For this review, take the finished solid that the model builds, in its own axes (mm). Give positions to 0.01 mm unless a question says otherwise; leave off trailing zeros. Loops run counter-clockwise (first coordinate to the right, second up) from the corner with the lowest first, then second, coordinate; pieces in that order, holes last.
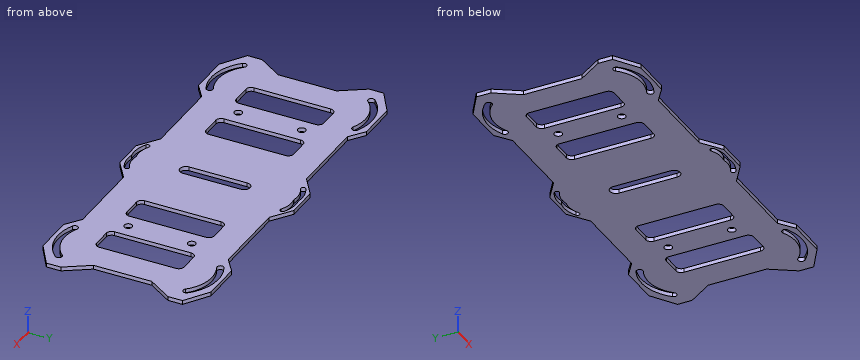
```python
from build123d import *

# Parameters (mm, degrees)
SCHIZZO1_R                   = 1.5
ESTRUSIONE_ESTRUSIONE1_DEPTH = 0.75


with BuildPart() as part:
    # Schizzo1 → Estrusione-Estrusione1 (new body, symmetric)
    with BuildSketch(Plane.XY):
        Polygon((-43.5, -27.5), (-13.615232638, -27.5), (-5.964504028, -32.859521299), (5.964504028, -32.859521299), (13.615232638, -27.5), (43.5, -27.5), (49.293787181, -31.722358535), (64.293787181, -31.722358535), (73.508072858, -25.714285677), (73.508072858, -20.214285677), (67.5, -11), (67.5, 11), (73.508072858, 20.214285677), (73.508072858, 25.714285677), (64.293787181, 31.722358535), (49.293787181, 31.722358535), (43.5, 27.5), (13.615232638, 27.5), (5.964504028, 32.859521299), (-5.964504028, 32.859521299), (-13.615232638, 27.5), (-43.5, 27.5), (-49.293787181, 31.722358535), (-64.293787181, 31.722358535), (-73.508072858, 25.714285677), (-73.508072858, 20.214285677), (-67.5, 11), (-67.5, -11), (-73.508072858, -20.214285677), (-73.508072858, -25.714285677), (-64.293787181, -31.722358535), (-49.293787181, -31.722358535), align=None)
        with BuildLine():
            ThreePointArc((-48.754479002, -28.623738791), (-59.172775767, -30.009764998), (-68.405644393, -24.988200197))
            ThreePointArc((-68.405644393, -24.988200197), (-68.356417198, -23.226138607), (-66.594355607, -23.275365801))
            ThreePointArc((-66.594355607, -23.275365801), (-58.719274878, -27.558458065), (-49.83309536, -26.376261209))
            ThreePointArc((-49.83309536, -26.376261209), (-48.17004839, -26.960691821), (-48.754479002, -28.623738791))
        make_face(mode=Mode.SUBTRACT)
        with Locations((-40.191447808, -12)):
            Circle(SCHIZZO1_R, mode=Mode.SUBTRACT)
        with BuildLine():
            ThreePointArc((0, -31.496185519), (-4.133745369, -31.563971562), (-8.018095478, -30.148249145))
            ThreePointArc((-8.018095478, -30.148249145), (-8.326872952, -28.953648185), (-7.132271992, -28.644870711))
            ThreePointArc((-7.132271992, -28.644870711), (-3.764579281, -29.856257566), (-0.187146253, -29.75240554))
            ThreePointArc((-0.187146253, -29.75240554), (0, -29.732097651), (0.187146253, -29.75240554))
            ThreePointArc((0.187146253, -29.75240554), (3.764579281, -29.856257566), (7.132271992, -28.644870711))
            ThreePointArc((7.132271992, -28.644870711), (8.326872952, -28.953648185), (8.018095478, -30.148249145))
            ThreePointArc((8.018095478, -30.148249145), (4.133745369, -31.563971562), (0, -31.496185519))
        make_face(mode=Mode.SUBTRACT)
        with BuildLine():
            ThreePointArc((66.594355607, -23.275365801), (68.356417198, -23.226138607), (68.405644393, -24.988200197))
            ThreePointArc((68.405644393, -24.988200197), (59.172775767, -30.009764998), (48.754479002, -28.623738791))
            ThreePointArc((48.754479002, -28.623738791), (48.17004839, -26.960691821), (49.83309536, -26.376261209))
            ThreePointArc((49.83309536, -26.376261209), (58.719274878, -27.558458065), (66.594355607, -23.275365801))
        make_face(mode=Mode.SUBTRACT)
        with Locations((40.191447808, -12)):
            Circle(SCHIZZO1_R, mode=Mode.SUBTRACT)
        with BuildLine():
            Line((-47.5, -16.5), (-54.5, -16.5))
            ThreePointArc((-54.5, -16.5), (-55.914213562, -15.914213562), (-56.5, -14.5))
            Line((-56.5, -14.5), (-56.5, 14.5))
            ThreePointArc((-56.5, 14.5), (-55.914213562, 15.914213562), (-54.5, 16.5))
            Line((-54.5, 16.5), (-47.5, 16.5))
            ThreePointArc((-47.5, 16.5), (-46.085786438, 15.914213562), (-45.5, 14.5))
            Line((-45.5, 14.5), (-45.5, -14.5))
            ThreePointArc((-45.5, -14.5), (-46.085786438, -15.914213562), (-47.5, -16.5))
        make_face(mode=Mode.SUBTRACT)
        with Locations((-40.191447808, 12)):
            Circle(SCHIZZO1_R, mode=Mode.SUBTRACT)
        with BuildLine():
            Line((-25.5, -16.5), (-32.5, -16.5))
            ThreePointArc((-32.5, -16.5), (-33.914213562, -15.914213562), (-34.5, -14.5))
            Line((-34.5, -14.5), (-34.5, 14.5))
            ThreePointArc((-34.5, 14.5), (-33.914213562, 15.914213562), (-32.5, 16.5))
            Line((-32.5, 16.5), (-25.5, 16.5))
            ThreePointArc((-25.5, 16.5), (-24.085786438, 15.914213562), (-23.5, 14.5))
            Line((-23.5, 14.5), (-23.5, -14.5))
            ThreePointArc((-23.5, -14.5), (-24.085786438, -15.914213562), (-25.5, -16.5))
        make_face(mode=Mode.SUBTRACT)
        with BuildLine():
            ThreePointArc((-2.261398956, 11), (0, 13.261398956), (2.261398956, 11))
            Line((2.261398956, 11), (2.261398956, -11))
            ThreePointArc((2.261398956, -11), (0, -13.261398956), (-2.261398956, -11))
            Line((-2.261398956, -11), (-2.261398956, 11))
        make_face(mode=Mode.SUBTRACT)
        with BuildLine():
            ThreePointArc((-66.594355607, 23.275365801), (-68.356417198, 23.226138607), (-68.405644393, 24.988200197))
            ThreePointArc((-68.405644393, 24.988200197), (-67.961138694, 25.440973547), (-67.5, 25.876794757))
            ThreePointArc((-67.5, 25.876794757), (-58.546813094, 30.113494239), (-48.754479002, 28.623738791))
            ThreePointArc((-48.754479002, 28.623738791), (-48.17004839, 26.960691821), (-49.83309536, 26.376261209))
            ThreePointArc((-49.83309536, 26.376261209), (-58.719274878, 27.558458065), (-66.594355607, 23.275365801))
        make_face(mode=Mode.SUBTRACT)
        with BuildLine():
            ThreePointArc((25.5, -16.5), (24.085786438, -15.914213562), (23.5, -14.5))
            Line((23.5, -14.5), (23.5, 14.5))
            ThreePointArc((23.5, 14.5), (24.085786438, 15.914213562), (25.5, 16.5))
            Line((25.5, 16.5), (32.5, 16.5))
            ThreePointArc((32.5, 16.5), (33.914213562, 15.914213562), (34.5, 14.5))
            Line((34.5, 14.5), (34.5, -14.5))
            ThreePointArc((34.5, -14.5), (33.914213562, -15.914213562), (32.5, -16.5))
            Line((32.5, -16.5), (25.5, -16.5))
        make_face(mode=Mode.SUBTRACT)
        with BuildLine():
            ThreePointArc((47.5, -16.5), (46.085786438, -15.914213562), (45.5, -14.5))
            Line((45.5, -14.5), (45.5, 14.5))
            ThreePointArc((45.5, 14.5), (46.085786438, 15.914213562), (47.5, 16.5))
            Line((47.5, 16.5), (54.5, 16.5))
            ThreePointArc((54.5, 16.5), (55.914213562, 15.914213562), (56.5, 14.5))
            Line((56.5, 14.5), (56.5, -14.5))
            ThreePointArc((56.5, -14.5), (55.914213562, -15.914213562), (54.5, -16.5))
            Line((54.5, -16.5), (47.5, -16.5))
        make_face(mode=Mode.SUBTRACT)
        with Locations((40.191447808, 12)):
            Circle(SCHIZZO1_R, mode=Mode.SUBTRACT)
        with BuildLine():
            ThreePointArc((0.187146253, 29.75240554), (0, 29.732097651), (-0.187146253, 29.75240554))
            ThreePointArc((-0.187146253, 29.75240554), (-3.764579281, 29.856257566), (-7.132271992, 28.644870711))
            ThreePointArc((-7.132271992, 28.644870711), (-8.326872952, 28.953648185), (-8.018095478, 30.148249145))
            ThreePointArc((-8.018095478, 30.148249145), (-4.133745369, 31.563971562), (0, 31.496185519))
            ThreePointArc((0, 31.496185519), (4.133745369, 31.563971562), (8.018095478, 30.148249145))
            ThreePointArc((8.018095478, 30.148249145), (8.326872952, 28.953648185), (7.132271992, 28.644870711))
            ThreePointArc((7.132271992, 28.644870711), (3.764579281, 29.856257566), (0.187146253, 29.75240554))
        make_face(mode=Mode.SUBTRACT)
        with BuildLine():
            ThreePointArc((48.754479002, 28.623738791), (59.172775767, 30.009764998), (68.405644393, 24.988200197))
            ThreePointArc((68.405644393, 24.988200197), (68.356417198, 23.226138607), (66.594355607, 23.275365801))
            ThreePointArc((66.594355607, 23.275365801), (58.719274878, 27.558458065), (49.83309536, 26.376261209))
            ThreePointArc((49.83309536, 26.376261209), (48.17004839, 26.960691821), (48.754479002, 28.623738791))
        make_face(mode=Mode.SUBTRACT)
    extrude(amount=ESTRUSIONE_ESTRUSIONE1_DEPTH, both=True)


solid = part.part
```
Item 1: Take a section at C-C on z = 0.2. State how many separate pieces and enclosed holes the cut face has, and give its area (3 significant figures).
Answer:
separate pieces: 1
enclosed holes: 15
area: 6,410 mm2
Item 2: Take a section at B-B on x = -21.5. Give the boundary of the cut face in (y, z).
Answer:
outline: (-27.5, -0.75) - (27.5, -0.75) - (27.5, 0.75) - (-27.5, 0.75) - close
Item 3: Clearance check with flat-ended pins moving along their axes: pin 1 Ø0.8 at (y, z) = (-2, 0) entering from +X; pin 2 Ø0.8 at (y, z) = (1, -0.5) entering from -X; pin 3 Ø2.5 at (x, y) = (-40.19, -12) entering from -Z; pin 4 Ø0.8 at (x, z) = (-52.5, 0) entering from -Y. State where each tip first meets the part, or that it passes through.
Answer:
pin 1: stops at x = 67.5
pin 2: stops at x = -67.5
pin 3: passes through
pin 4: stops at y = -31.72
Item 4: Take a section at A-A on y = 0.5. Give the boundary of the cut face in (x, z).
Answer:
outline: (-67.5, -0.75) - (-56.5, -0.75) - (-56.5, 0.75) - (-67.5, 0.75) - close; (-45.5, -0.75) - (-34.5, -0.75) - (-34.5, 0.75) - (-45.5, 0.75) - close; (-23.5, -0.75) - (-2.26, -0.75) - (-2.26, 0.75) - (-23.5, 0.75) - close; (2.26, -0.75) - (23.5, -0.75) - (23.5, 0.75) - (2.26, 0.75) - close; (34.5, -0.75) - (45.5, -0.75) - (45.5, 0.75) - (34.5, 0.75) - close; (56.5, -0.75) - (67.5, -0.75) - (67.5, 0.75) - (56.5, 0.75) - close
Item 5: For L1, parallel to X at y = 2, z = -0.55; L2, parallel to Y at x = -28, z = -0.5; L3, parallel to X at y = -14, z = 0.4, list the stretches that pass through material, from the lowest coordinate up.
Answer:
L1: x = -67.5 to -56.5, -45.5 to -34.5, -23.5 to -2.26, 2.26 to 23.5, 34.5 to 45.5, 56.5 to 67.5
L2: y = -27.5 to -16.5, 16.5 to 27.5
L3: x = -69.46 to -56.5, -45.5 to -34.5, -23.5 to 23.5, 34.5 to 45.5, 56.5 to 69.46
